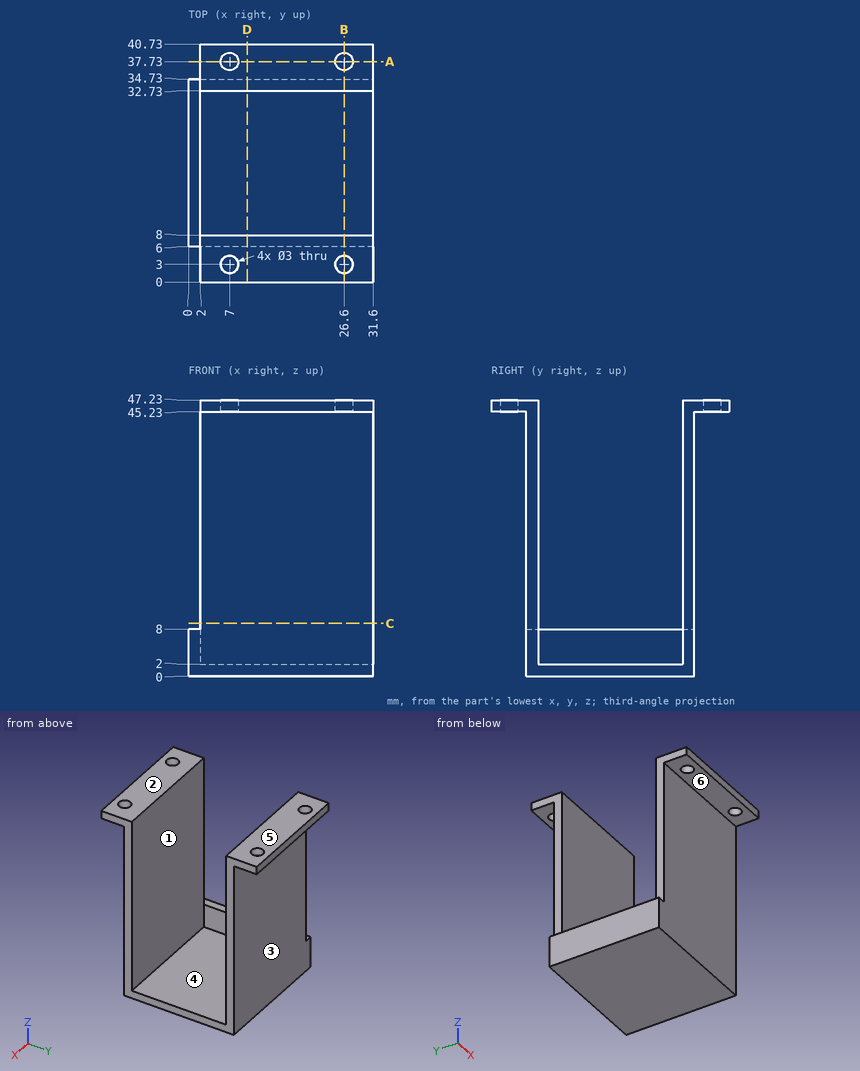
The drawing under review shows one solid part. Ordinate dimensions are in mm from its lowest x, y, z. A direction names the side the tool comes from. Give positions to 0.01 mm unless a question says otherwise; leave off trailing zeros. Order: outer loops, then holes, each group sorted by start corner. A loop starts at its lowest first (then second) coordinate and runs counter-clockwise, first axis right, second up. Notation, with made-up numbers: M 5.25,81 L 50.25,81 A8 cw 50.25,91 Z; hole C 35.25,19.25 d1. An arc over 180 degrees is marked long. One line per question, with ' | ' between items. Start each with the question number.
Q1. For L1, parallel to Y at x = 7, z = 46.4; L2, parallel to X at y = 3, z = 46; L3, parallel to Y at x = 23.5, z = 39.5, list the stretches that pass through material, from the lowest coordinate up. Write a range as [from, to].
Q2. We need section D-D (x = 10). Write out the cut boundary in (y, z).
Q3. For pin 1 Ø6 at (x, y) = (8.5, 16.5) entering from +Z; pin 2 Ø1.8 at (x, y) = (11, 2.5) entering from -Z; pin 3 Ø0.6 at (x, y) = (1, 15.5) entering from +Z; pin 4 Ø10 at (y, z) = (17, 24) entering from -X, all flat-tipped, find the tip position at first contact; note any pin that passes through.
Q4. We need section B-B (x = 26.6). Write out the cut boundary in (y, z).
Q5. We need section C-C (z = 9). Write out the cut boundary in (x, y), plus the area to 3 significant figures.
Q6. The part is to be moulded in two halves that separate along Y. For the marked faces 1, 2 and 3, say which applies: +Y half, -Y half, draft (parallel to the pull), parting line (faces both ways), or undercut.
Q7. Machinability: for the marked faces 4, 5 and 6, which of the approach directions +Z, -Z, +X, -X, +Y, -Y give a long, thin tool a straight path to every point of the face, cutting with its end or side? Answer none if there is none.
Q8. We need section A-A (y = 37.73). Write out the cut boundary in (x, z).
Returned:
1) L1: [0, 1.5], [4.5, 8], [32.73, 36.23], [39.23, 40.73] | L2: [2, 5.5], [8.5, 25.1], [28.1, 31.6] | L3: [6, 8], [32.73, 34.73]
2) outline: M 0,45.23 L 6,45.23 L 6,0 L 34.73,0 L 34.73,45.23 L 40.73,45.23 L 40.73,47.23 L 32.73,47.23 L 32.73,2 L 8,2 L 8,47.23 L 0,47.23 Z
3) pin 1: z = 2 | pin 2: z = 45.23 | pin 3: z = 8 | pin 4: through
4) outline: M 0,45.23 L 1.5,45.23 L 1.5,47.23 L 0,47.23 Z; M 4.5,45.23 L 6,45.23 L 6,0 L 34.73,0 L 34.73,45.23 L 36.23,45.23 L 36.23,47.23 L 32.73,47.23 L 32.73,2 L 8,2 L 8,47.23 L 4.5,47.23 Z; M 39.23,45.23 L 40.73,45.23 L 40.73,47.23 L 39.23,47.23 Z
5) outline: M 2,6 L 31.6,6 L 31.6,8 L 2,8 Z; M 2,32.73 L 31.6,32.73 L 31.6,34.73 L 2,34.73 Z | area: 118 mm2
6) face 1: undercut | face 2: draft | face 3: +Y half
7) face 4: +Z, +X | face 5: +Z, +X, -X, +Y, -Y | face 6: -Z, +X, -X, -Y
8) outline: M 2,45.23 L 5.5,45.23 L 5.5,47.23 L 2,47.23 Z; M 8.5,45.23 L 25.1,45.23 L 25.1,47.23 L 8.5,47.23 Z; M 28.1,45.23 L 31.6,45.23 L 31.6,47.23 L 28.1,47.23 Z
